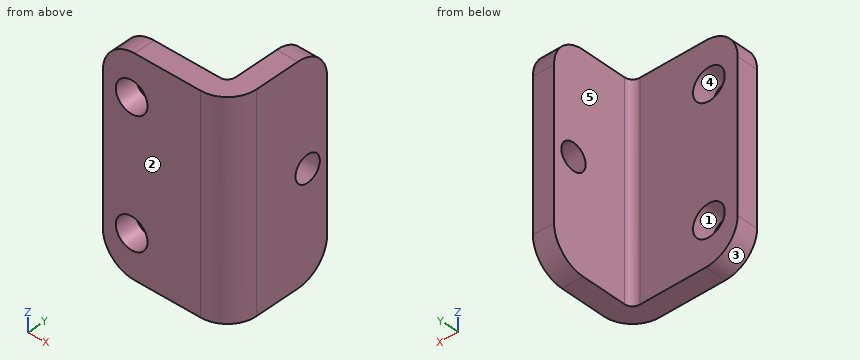
```python
from build123d import *

# Parameters (mm, degrees)
SKETCH1_R                    = 1.5
BASE_FLANGE1_DEPTH           = 2
EDGE_FLANGE1_STRIP_W         = 9.5
EDGE_FLANGE1_STRIP_H         = 2
EDGE_FLANGE1_STRIP_CUT_DEPTH = 20
EDGE_FLANGE1_DEPTH           = 20
SKETCH9_R                    = 1.25
CUT_EXTRUDE1_DEPTH           = 10
FILLET1_R                    = 3


# Sheet-metal steps are written as plain solids
with BuildPart() as part:
    # Sketch1 → Base-Flange1 (new body)
    with BuildSketch(Plane(origin=(0, 0, 0), x_dir=(1, 0, 0), z_dir=(0, 1, 0))):
        with BuildLine():
            Line((0, 7), (0, -7))
            ThreePointArc((0, -7), (0.878679656, -9.121320344), (3, -10))
            Line((3, -10), (12, -10))
            Line((12, -10), (12, 10))
            Line((12, 10), (3, 10))
            ThreePointArc((3, 10), (0.878679656, 9.121320344), (0, 7))
        make_face()
        with Locations(Location((2.72, 6, 0), (0, 0, 270))):
            Circle(SKETCH1_R, mode=Mode.SUBTRACT)
        with Locations(Location((2.72, -6, 0), (0, 0, 270))):
            Circle(SKETCH1_R, mode=Mode.SUBTRACT)
    extrude(amount=BASE_FLANGE1_DEPTH)

    # Edge-Flange1 strip (across the edge) → Edge-Flange1 strip cut (cut)
    with BuildSketch(Plane(origin=(12, 2, 10), x_dir=(-1, 0, 0), z_dir=(0, 0, -1))):
        with Locations((-2, -1)):
            Rectangle(EDGE_FLANGE1_STRIP_W, EDGE_FLANGE1_STRIP_H)
    extrude(amount=EDGE_FLANGE1_STRIP_CUT_DEPTH, mode=Mode.SUBTRACT)

    # Edge-Flange1 section (across the edge) → Edge-Flange1 (add)
    with BuildSketch(Plane(origin=(12, 2, 10), x_dir=(-1, 0, 0), z_dir=(0, 0, -1))):
        with BuildLine():
            Line((0, 0.75), (0, 8))
            Line((0, 8), (2, 8))
            Line((2, 8), (2, 0.75))
            ThreePointArc((2, 0.75), (2.219669914, 0.219669914), (2.75, 0))
            Line((2.75, 0), (2.75, -2))
            ThreePointArc((2.75, -2), (0.805456352, -1.194543648), (0, 0.75))
        make_face()
    extrude(amount=EDGE_FLANGE1_DEPTH)

    # Sketch9 → Cut-Extrude1 (cut)
    with BuildSketch(Plane.ZY.offset(-10)):
        with Locations(Location((0, 8, 0), (0, 0, 270))):
            Circle(SKETCH9_R)
    extrude(amount=-CUT_EXTRUDE1_DEPTH, mode=Mode.SUBTRACT)

    # Fillet1
    fillet1_edges = [part.edges().sort_by_distance(p)[0] for p in [
        (11, 10, 10),
        (11, 10, -10),
    ]]
    fillet(fillet1_edges, radius=FILLET1_R)


solid = part.part
```
For this review, take the finished solid that the model builds, in its own axes (mm). Face numbers are marked on the shaded views. A direction names the side the tool comes from. Coordinates: 2 decimals unless noted, no trailing zeros. Write each loop counter-clockwise with the first axis right and the second up, starting at its lowest first coordinate (ties: lowest second). Pieces come first, ordered by that corner, then holes.
(1) Add section D-D on z = -3.5. Give the boundary of the cut face in (x, y).
(2) Wall thickness on probe 1 along Y at (x, z) = (7.5, 5.25); probe 2 along X at (y, z) = (1.2, 6); probe 3 along X at (y, z) = (0.85, 6): over which ranges is each line inside the solid? List them lowest first.
(3) Add section A-A on z = -6. Give the boundary of the cut face in (x, y), then the cut area to 3 significant figures.
(4) The part is to be moulded in two halves that separate along X. For the marked faces 1, 2 and 3, say which applies: +X half, -X half, draft (parallel to the pull), parting line (faces both ways), or undercut.
(5) Tool access review of the marked faces 4 and 5: name each direction out of +Z, -Z, +X, -X, +Y, -Y from which nothing blocks a thin tool from reaching the whole face with its end or side.
(6) For pin 1 Ø2 at (y, z) = (4.5, -1) entering from -X; pin 2 Ø6 at (x, y) = (2.5, 3.5) entering from -Z; pin 3 Ø1 at (x, y) = (10.5, 8.5) entering from +Z, all flat-tipped, find the tip position at first contact; note any pin that passes through.
(7) Add section B-B on x = 2.72. Give the boundary of the cut face in (y, z).
(8) Add section C-C on y = 8. Give the boundary of the cut face in (x, z), then the cut area to 3 significant figures.
Answer sheet:
1. outline: (0, 0) - (9.25, 0) arc R2.75 ccw to (12, 2.75) - (12, 10) - (10, 10) - (10, 2.75) arc R0.75 cw to (9.25, 2) - (0, 2) - close
2. probe 1: y = 0 to 2
2. probe 2: x = 0 to 1.22, 4.22 to 11.52
2. probe 3: x = 0 to 1.22, 4.22 to 11.24
3. outline: (0, 0) - (1.22, 0) - (1.22, 2) - (0, 2) - close; (4.22, 0) - (9.25, 0) arc R2.75 ccw to (12, 2.75) - (12, 10) - (10, 10) - (10, 2.75) arc R0.75 cw to (9.25, 2) - (4.22, 2) - close
3. area: 32.5 mm2
4. face 1: undercut
4. face 2: draft
4. face 3: -X half
5. face 4: +Y, -Y
5. face 5: +Z, -Z, -X, +Y
6. pin 1: stops at x = 10
6. pin 2: stops at z = -10
6. pin 3: stops at z = 9.83
7. outline: (0, -9.99) - (2, -9.99) - (2, -7.5) - (0, -7.5) - close; (0, -4.5) - (2, -4.5) - (2, 4.5) - (0, 4.5) - close; (0, 7.5) - (2, 7.5) - (2, 9.99) - (0, 9.99) - close
8. outline: (10, -9.83) - (12, -9.83) - (12, -1.25) - (10, -1.25) - close; (10, 1.25) - (12, 1.25) - (12, 9.83) - (10, 9.83) - close
8. area: 34.3 mm2
